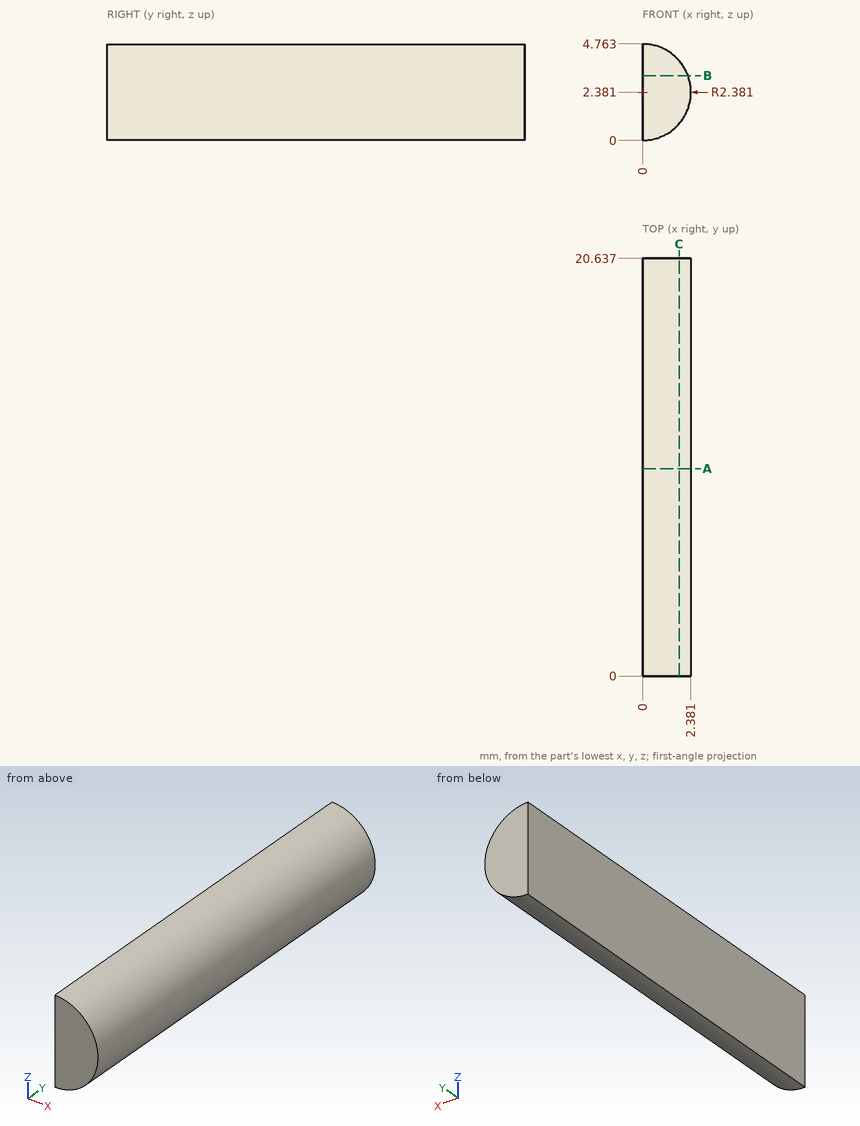
Here's the drawing with two shaded views (mm, measured from the low corner). I have some questions. Give positions to 0.01 mm unless a question says otherwise; leave off trailing zeros. Write each loop counter-clockwise with the first axis right and the second up, starting at its lowest first coordinate (ties: lowest second). Pieces come first, ordered by that corner, then holes. Notation, with made-up numbers: (52, -26) -> (68, -26) arc R15 cw to (68, -9) -> close; hole circle Ø7 at (27.5, -6). An arc over 180 degrees is marked (long way). Use one line per item in the form item = value. Start each with the question number.
1. Imagine slicing it at C-C on x = 1.8. List the corners of the cut face in (y, z) for me.
2. If I drill on L1, parallel to X at y = 5, z = 2.25; L2, parallel to Z at x = 1.55, y = 10.5 (1 decimal); L3, parallel to Z at x = 0.85, y = 10.75 (1 decimal), over which ranges is the centre line in solid material (lowest first)?
3. Imagine slicing it at A-A on y = 10.25. List the corners of the cut face in (x, z) for me.
4. Imagine slicing it at B-B on z = 3.2. List the corners of the cut face in (x, y) for me.
5. Will this pin go through, and if not, where does the flat tip stop? pin 1 Ø1 at (x, y) = (1.5, 13.5) entering from +Z.
Entries:
q1.outline = (0, 0.82) -> (20.64, 0.82) -> (20.64, 3.94) -> (0, 3.94) -> close
q2.L1 = 0 to 2.38
q2.L2 = 0.6 to 4.2
q2.L3 = 0.2 to 4.6
q3.outline = (0, 0) arc R2.38 ccw to (0, 4.76) -> close
q4.outline = (0, 0) -> (2.24, 0) -> (2.24, 20.64) -> (0, 20.64) -> close
q5.pin_1 = 4.54
